from build123d import *

# Parameters (mm, degrees)
ESBO_O1_W                  = 26
ESBO_O1_H                  = 34
RESSALTO_EXTRUS_O1_DEPTH   = 10
CHANFRO2_SIZE              = 1.4
CORTE_EXTRUS_O1_DEPTH      = 24.622023622
CORTE_EXTRUS_O1_DEPTH_BACK = 24.622023622
ESBO_O8_R                  = 1.35
CORTE_EXTRUS_O2_DEPTH      = 10
ESBO_O9_R                  = 1.025
CORTE_EXTRUS_O3_DEPTH      = 10
ESBO_O11_R                 = 1.35
CORTE_EXTRUS_O5_DEPTH      = 4


with BuildPart() as part:
    # Esboço1 → Ressalto-extrusão1 (new body)
    with BuildSketch(Plane.XY):
        Rectangle(ESBO_O1_W, ESBO_O1_H)
    extrude(amount=RESSALTO_EXTRUS_O1_DEPTH)

    # Chanfro2
    chanfro2_edges = [part.edges().sort_by_distance(p)[0] for p in [
        (0, -17, 0),
    ]]
    chamfer(chanfro2_edges, length=CHANFRO2_SIZE)

    # Esboço5 → Corte-extrusão1 (cut, two sides: drawn at the far end of the back side and taken through both)
    with BuildSketch(Plane(origin=(0, 0, 0), x_dir=(0, 0, -1), z_dir=(1, 0, 0)).offset(-CORTE_EXTRUS_O1_DEPTH_BACK)):
        Polygon((0, 17), (-10, 17), (-10, 10.5380702), align=None)
    extrude(amount=CORTE_EXTRUS_O1_DEPTH + CORTE_EXTRUS_O1_DEPTH_BACK, mode=Mode.SUBTRACT)

    # Esboço8 → Corte-extrusão2 (cut)
    with BuildSketch(Plane(origin=(13, 0, 0), x_dir=(0, 0, -1), z_dir=(1, 0, 0))):
        with Locations((-2.8, 8.5)):
            Circle(ESBO_O8_R)
        with Locations((-2.8, -13.5)):
            Circle(ESBO_O8_R)
    extrude(amount=-CORTE_EXTRUS_O2_DEPTH, mode=Mode.SUBTRACT)

    # Esboço9 → Corte-extrusão3 (cut)
    with BuildSketch(Plane.ZY.offset(13)):
        with Locations((2.8, 8.5)):
            Circle(ESBO_O9_R)
        with Locations((2.8, -13.5)):
            Circle(ESBO_O9_R)
    extrude(amount=-CORTE_EXTRUS_O3_DEPTH, mode=Mode.SUBTRACT)

    # Esboço11 → Corte-extrusão5 (cut)
    with BuildSketch(Plane.XY.offset(10)):
        with Locations((7, 0)):
            Circle(ESBO_O11_R)
        with Locations((0, -7)):
            Circle(ESBO_O11_R)
        with Locations((-7, 0)):
            Circle(ESBO_O11_R)
        with Locations((0, 7)):
            Circle(ESBO_O11_R)
    extrude(amount=-CORTE_EXTRUS_O5_DEPTH, mode=Mode.SUBTRACT)


solid = part.part
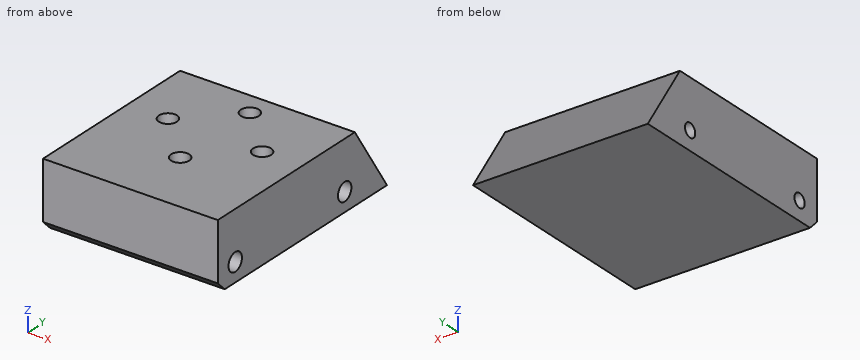
Verification items for the finished model (mm, model axes). Coordinates: 2 decimals unless noted, no trailing zeros. Order: outer loops, then holes, each group sorted by start corner. A loop starts at its lowest first (then second) coordinate and runs counter-clockwise, first axis right, second up. Notation, with made-up numbers: (-19, 46.5) -> (-9, 46.5) arc R18 ccw to (-9, 81.5) -> close; hole circle Ø7 at (-13, 28). An arc over 180 degrees is marked (long way). Put each result on its own line as item: value. Start each with the question number.
1. Cross-section at B-B, the plane z = 9. Record the boundary of the cut face in (x, y).
2. Cross-section at A-A, the plane x = -3.75. Record the boundary of the cut face in (y, z) (3 decimals).
3. Material ranges on L1, parallel to Y at x = -6.75, z = 2.8 (3 decimals); L2, parallel to Y at x = 9.25, z = 2.8; L3, parallel to Z at x = 9, y = 7.5, recorded low to high. Write a range as [from, to].
4. Cross-section at C-C, the plane y = 0. Record the boundary of the cut face in (x, z), then the cut area to 3 significant figures.
5. Go/stop test with flat-tipped pins: pin 1 Ø3.5 at (x, y) = (0, 7) entering from +Z; pin 2 Ø5 at (x, z) = (-10, 8.5) entering from +Y; pin 3 Ø1 at (y, z) = (-13.5, 2.5) entering from -X; pin 4 Ø1.6 at (y, z) = (8.5, 2.8) entering from +X. Record where each tip stops, or that it passes through.
6. Cross-section at D-D, the plane x = 2. Record the boundary of the cut face in (y, z), then the cut area to 3 significant figures.
Computed:
1. outline: (-13, -17) -> (13, -17) -> (13, 11.18) -> (-13, 11.18) -> close; hole circle Ø2.7 at (-7, 0); hole circle Ø2.7 at (0, -7); hole circle Ø2.7 at (0, 7); hole circle Ø2.7 at (7, 0)
2. outline: (-17, 1.4) -> (-15.6, 0) -> (17, 0) -> (10.538, 10) -> (-17, 10) -> close; hole circle Ø2.05 at (-13.5, 2.8); hole circle Ø2.05 at (8.5, 2.8)
3. L1: [-17, -14.525], [-12.475, 7.475], [9.525, 15.191]
3. L2: [-17, -14.85], [-12.15, 7.15], [9.85, 15.19]
3. L3: [0, 1.89], [3.71, 10]
4. outline: (-13, 0) -> (13, 0) -> (13, 10) -> (8.35, 10) -> (8.35, 6) -> (5.65, 6) -> (5.65, 10) -> (-5.65, 10) -> (-5.65, 6) -> (-8.35, 6) -> (-8.35, 10) -> (-13, 10) -> close
4. area: 238 mm2
5. pin 1: z = 10
5. pin 2: y = 13.12
5. pin 3: x = -3
5. pin 4: x = 3
6. outline: (-17, 1.4) -> (-15.6, 0) -> (17, 0) -> (10.54, 10) -> (-17, 10) -> close
6. area: 307 mm2
